Part print with two shaded views. Sizes in mm from the minimum x, y, z corner. A direction names the side the tool comes from. Round coordinates to 2 decimals unless told otherwise and drop trailing zeros. Write each loop counter-clockwise with the first axis right and the second up, starting at its lowest first coordinate (ties: lowest second). Pieces come first, ordered by that corner, then holes. Notation, with made-up numbers: (50, -22) -> (60, -22) arc R23 ccw to (60, 11) -> close; hole circle Ø6 at (80, -23). An arc over 180 degrees is marked (long way). Return JSON: item names as keys, results as strings. Group by question number.
(1) Tool access for the marked faces 5, 6, 7 and 8: list every direction of +Z, -Z, +X, -X, +Y, -Y with a clear straight run to the whole face (end or side of a thin tool).
(2) Drop flat-ended pins along their axis: pin 1 Ø10 at (y, z) = (29.5, 9) entering from -X; pin 2 Ø10 at (x, z) = (15.5, 21.5) entering from +Y; pin 3 Ø3 at (x, y) = (29, 16) entering from +Z; pin 4 Ø3 at (x, z) = (47.5, 4.5) entering from +Y. Give the stop position or say it passes through.
(3) Drill centre lines: L1, parallel to Z at x = 55, y = 4.25; L2, parallel to X at y = 34, z = 20; L3, parallel to X at y = 7, z = 25. Where is each one in solid material? Low to high. Write a range as from..to.
(4) Saw through at B-B (z = 8.5). List the corners of the cut face in (x, y).
(5) Saw through at A-A (y = 37). List the corners of the cut face in (x, z).
(6) Saw through at C-C (y = 7). List the corners of the cut face in (x, z).
(7) Mould opens along X. For the marked faces 1, 2, 3 and 4 say: +X half, -X half, draft (parallel to the pull), parting line (faces both ways), or undercut.
(8) Saw through at D-D (x = 37.5). List the corners of the cut face in (y, z), plus the area to 3 significant figures.
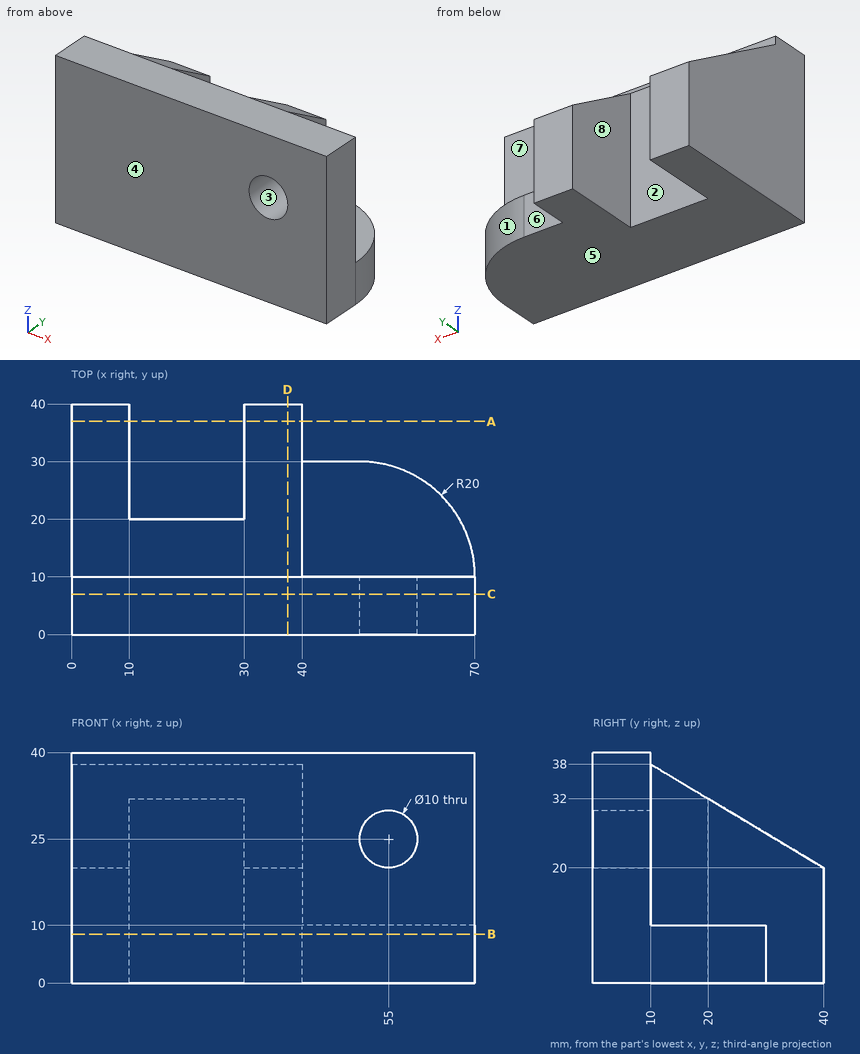
Computed values:
{
 "1": {"face 5": "-Z, +X, -X, +Y, -Y", "face 6": "+Z, -Z, +X, +Y", "face 7": "+Z, +X, +Y", "face 8": "+Z, -Z, +Y"},
 "2": {"pin 1": "x = 0", "pin 2": "y = 20", "pin 3": "z = 35.3", "pin 4": "y = 30"},
 "3": {"L1": "0..20, 30..40", "L2": "0..10, 30..40", "L3": "0..50, 60..70"},
 "4": {"outline": "(0, 0) -> (70, 0) -> (70, 10) arc R20 ccw to (50, 30) -> (40, 30) -> (40, 40) -> (30, 40) -> (30, 20) -> (10, 20) -> (10, 40) -> (0, 40) -> close"},
 "5": {"outline": "(0, 0) -> (10, 0) -> (10, 21.8) -> (0, 21.8) -> close; (30, 0) -> (40, 0) -> (40, 21.8) -> (30, 21.8) -> close"},
 "6": {"outline": "(0, 0) -> (70, 0) -> (70, 40) -> (0, 40) -> close; hole circle Ø10 at (55, 25)"},
 "7": {"face 1": "+X half", "face 2": "undercut", "face 3": "undercut", "face 4": "draft"},
 "8": {"outline": "(0, 0) -> (40, 0) -> (40, 20) -> (10, 38) -> (10, 40) -> (0, 40) -> close", "area": "1,270 mm2"}
}
